from build123d import *

# Parameters (mm, degrees)
SKETCH1_R               = 14.2875
BOSS_EXTRUDE1_DEPTH     = 76.2
SKETCH2_W               = 25.4
SKETCH2_H               = 50.8
SKETCH2_W_2             = 104.590829903
SKETCH2_W_3             = 68.699540571
SKETCH2_R               = 2.5
CUT_EXTRUDE1_DEPTH      = 1
CUT_EXTRUDE1_DEPTH_BACK = 39.1


with BuildPart() as part:
    # Sketch1 → Boss-Extrude1 (new body)
    with BuildSketch(Plane(origin=(0, 0, 0), x_dir=(1, 0, 0), z_dir=(0, 1, 0))):
        with BuildLine():
            Line((63.5, 0), (-63.5, 0))
            ThreePointArc((-63.5, 0), (-76.970384182, -32.520384182), (-44.45, -19.05))
            ThreePointArc((-44.45, -19.05), (-42.743933719, -12.807304268), (-38.1, -8.3))
            Line((-38.1, -8.3), (38.1, -8.3))
            ThreePointArc((38.1, -8.3), (42.743933719, -12.807304268), (44.45, -19.05))
            ThreePointArc((44.45, -19.05), (76.970384182, -32.520384182), (63.5, 0))
        make_face()
        with Locations((-63.5, -19.05)):
            Circle(SKETCH1_R, mode=Mode.SUBTRACT)
        with Locations((63.5, -19.05)):
            Circle(SKETCH1_R, mode=Mode.SUBTRACT)
    extrude(amount=BOSS_EXTRUDE1_DEPTH)

    # Sketch2 → Cut-Extrude1 (cut, two sides)
    with BuildSketch(Plane(origin=(0, 0, 0), x_dir=(-1, 0, 0), z_dir=(0, 0, -1))) as cut_extrude1_sk:
        with Locations((-50.8, 38.1)):
            Rectangle(SKETCH2_W, SKETCH2_H)
        with Locations((-115.795414952, 38.1)):
            Rectangle(SKETCH2_W_2, SKETCH2_H)
        with Locations((50.8, 38.1)):
            Rectangle(SKETCH2_W, SKETCH2_H)
        with Locations((97.849770285, 38.1)):
            Rectangle(SKETCH2_W_3, SKETCH2_H)
        with Locations((-15.500122677, 64.947)):
            Circle(SKETCH2_R)
        with Locations((-15.500122677, 11.253)):
            Circle(SKETCH2_R)
        with Locations((31.000245354, 38.1)):
            Circle(SKETCH2_R)
    extrude(amount=CUT_EXTRUDE1_DEPTH, mode=Mode.SUBTRACT)
    extrude(cut_extrude1_sk.sketch, amount=-CUT_EXTRUDE1_DEPTH_BACK, mode=Mode.SUBTRACT)


solid = part.part
Design review of the part built by this model. Coordinates are the model's own, in mm. A direction names the side the tool comes from. Give positions to 0.01 mm unless a question says otherwise; leave off trailing zeros. Loops run counter-clockwise (first coordinate to the right, second up) from the corner with the lowest first, then second, coordinate; pieces in that order, holes last. Notation, with made-up numbers: (28, 12) - (77, 12) arc R31 cw to (77, 51) - close; hole circle Ø1 at (-13, 44.5). An arc over 180 degrees is marked (long way). Write item = value, one per line.
1) Take a section at C-C on x = -68. State the section outline as (y, z) points, and give its area (3 significant figures).
Result sheet:
outline = (0, 0.54) - (12.7, 0.54) - (12.7, 5.49) - (0, 5.49) - close; (0, 32.61) - (12.7, 32.61) - (12.7, 37.56) - (0, 37.56) - close; (63.5, 0.54) - (76.2, 0.54) - (76.2, 5.49) - (63.5, 5.49) - close; (63.5, 32.61) - (76.2, 32.61) - (76.2, 37.56) - (63.5, 37.56) - close
area = 251 mm2
2) To check wall thickness, follow line 1 (X direction, y = 70, z = 19); line 2 (Z direction, x = 63.5, y = 73.25); line 3 (Y direction, x = -43.5, z = 5). State the ranges of each line that lie inside material, in increasing order.
Result sheet:
line_1 = -82.55 to -77.79, -49.21 to -44.45, 44.45 to 49.21, 77.79 to 82.55
line_2 = 0 to 4.76, 33.34 to 38.1
line_3 = 0 to 12.7, 63.5 to 76.2
3) Draft analysis for pull direction X (two halves, no side actions). For faces 1 (the face through (-30.46, 35.66, 4.09)), 2 (the face through (0, 76.2, 8)), 3 (the face through (-38.1, 38, 4)), state which applies: +X half, -X half, draft (parallel to the pull), parting line (faces both ways), or undercut.
Result sheet:
face_1 = undercut
face_2 = draft
face_3 = -X half
4) Clearance check with flat-ended pins moving along their axes: pin 1 Ø4 at (x, y) = (15.5, 64.95) entering from -Z; pin 2 Ø6 at (x, y) = (-10, 62) entering from -Z; pin 3 Ø9 at (y, z) = (42.5, 4.5) entering from +X; pin 4 Ø9 at (y, z) = (48.5, 5.5) entering from -X. State where each tip first meets the part, or that it passes through.
Result sheet:
pin_1 = through
pin_2 = 0
pin_3 = 38.1
pin_4 = -38.1
5) Take a section at B-B on y = 38.1. State the section outline as (x, z) points.
Result sheet:
outline = (-38.1, 0) - (-33.5, 0) - (-33.5, 8.3) - (-38.1, 8.3) - close; (-28.5, 0) - (38.1, 0) - (38.1, 8.3) - (-28.5, 8.3) - close
6) Take a section at A-A on y = 6.5. Count the separate pieces of the cut face and the enclosed holes in it, and give its area (3 significant figures).
Result sheet:
separate_pieces = 1
enclosed_holes = 2
area = 1,930 mm2
7) Tool access review of faces 4 (the face through (-55, 12.7, 6)), 5 (the face through (-42.8, 69.8, 12.9)), 6 (the face through (-77.774, 69.761, 18.422)): name each direction out of +Z, -Z, +X, -X, +Y, -Y from which nothing blocks a thin tool from reaching the whole face with its end or side.
Result sheet:
face_4 = +Z, -Z, -X
face_5 = +Z, +Y, -Y
face_6 = +Y, -Y
